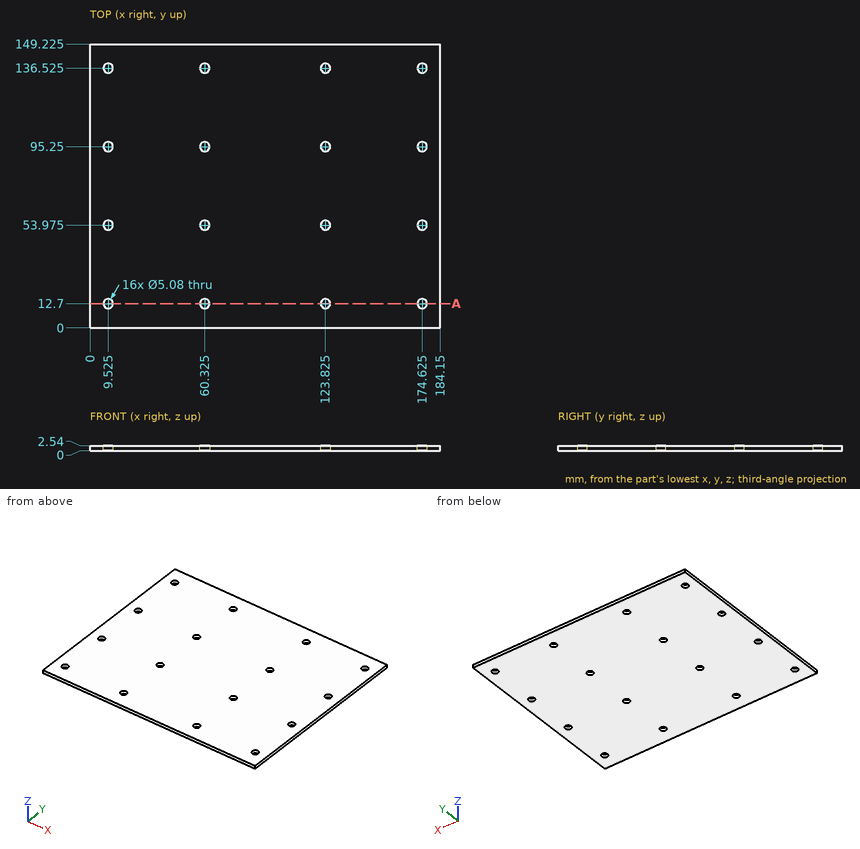
Could you check a few things on this drawing? It's one solid part, dimensions in mm from its lowest x, y, z. Round coordinates to 2 decimals unless told otherwise and drop trailing zeros. Loops run counter-clockwise (first coordinate to the right, second up) from the corner with the lowest first, then second, coordinate; pieces in that order, holes last. Notation, with made-up numbers: (46.5, 23.25) -> (76.5, 23.25) arc R7 ccw to (76.5, 34.25) -> close; hole circle Ø4 at (71.25, 71.25). An arc over 180 degrees is marked (long way). Answer as CSV lines item,"result".
1. If I drill on L1, parallel to Y at x = 175, z = 1.6 (3 decimals); L2, parallel to X at y = 95, z = 1.95; L3, parallel to Y at x = 61, z = 0.5 (3 decimals), over which ranges is the centre line in solid material (lowest first)?
Final values:
L1,"y = 0 to 10.188, 15.212 to 51.463, 56.487 to 92.738, 97.762 to 134.013, 139.037 to 149.225"
L2,"x = 0 to 7, 12.05 to 57.8, 62.85 to 121.3, 126.35 to 172.1, 177.15 to 184.15"
L3,"y = 0 to 10.251, 15.149 to 51.526, 56.424 to 92.801, 97.699 to 134.076, 138.974 to 149.225"
2. If we section it at A-A on y = 12.7: Please give me the cut outline in (x, z) (3 decimals), plus the area to 3 significant figures.
Final values:
outline,"(0, 0) -> (6.985, 0) -> (6.985, 2.54) -> (0, 2.54) -> close; (12.065, 0) -> (57.785, 0) -> (57.785, 2.54) -> (12.065, 2.54) -> close; (62.865, 0) -> (121.285, 0) -> (121.285, 2.54) -> (62.865, 2.54) -> close; (126.365, 0) -> (172.085, 0) -> (172.085, 2.54) -> (126.365, 2.54) -> close; (177.165, 0) -> (184.15, 0) -> (184.15, 2.54) -> (177.165, 2.54) -> close"
area,"416 mm^2"
3. For pin 1 (8 mm diameter, centred on x = 174.625, y = 136.525, fed in from +Z), with a flat end and sliding along its axis, tell me the tip position at first contact or that it passes through.
Final values:
pin 1,"stops at z = 2.54"
